Check sheet for the modelled part. Datum: model origin and axes. Units: mm. Face numbers are marked on the shaded views. A direction names the side the tool comes from. Coordinates: 2 decimals unless noted, no trailing zeros. Loops run counter-clockwise (first coordinate to the right, second up) from the corner with the lowest first, then second, coordinate; pieces in that order, holes last. Notation, with made-up numbers: M 81.25,55.25 L 98.25,55.25 A18 cw 98.25,68.25 Z; hole C -15,7 d5. An arc over 180 degrees is marked long. Return JSON: item names as keys, results as strings.
from build123d import *

# Parameters (mm, degrees)
SKETCH1_W                = 57.629592668
SKETCH1_H                = 21.211867522
SKETCH1_R                = 1.75
SKETCH1_R_2              = 4.5
BOSS_EXTRUDE1_DEPTH      = 6
SKETCH1_22_W             = 8.129592668
SKETCH1_22_H             = 21.211867522
SKETCH1_22_R             = 1.5
BOSS_EXTRUDE2_DEPTH      = 2
BOSS_EXTRUDE3_DEPTH      = 50.8
BOSS_EXTRUDE3_DEPTH_BACK = 50.8
SKETCH1_23_W             = 5
SKETCH1_23_H             = 75.291254256
SKETCH1_23_H_2           = 26.308745744
SKETCH4_W                = 57.748953374
SKETCH4_H                = 6
BOSS_EXTRUDE4_DEPTH      = 3
FILLET2_R                = 5
FILLET2_OF_MIRROR1_R     = 5


with BuildPart() as part:
    # Sketch1 → Boss-Extrude1 (new body)
    with BuildSketch(Plane(origin=(0, 0, 0), x_dir=(1, 0, 0), z_dir=(0, 1, 0))):
        with BuildLine():
            Line((-197.556308439, -13.154372872), (0, -13.154372872))
            ThreePointArc((0, -13.154372872), (13.154372872, 0), (0, 13.154372872))
            Line((0, 13.154372872), (-197.556308439, 13.154372872))
            Line((-197.556308439, 13.154372872), (-197.556308439, -13.154372872))
        make_face()
        with Locations((-104.57172107, -0.139435446)):
            Rectangle(SKETCH1_W, SKETCH1_H, mode=Mode.SUBTRACT)
        with Locations(Location((0, 8, 0), (0, 0, 270))):
            Circle(SKETCH1_R, mode=Mode.SUBTRACT)
        with Locations(Location((0, -8, 0), (0, 0, 270))):
            Circle(SKETCH1_R, mode=Mode.SUBTRACT)
        with Locations(Location((-8, 0, 0), (0, 0, 270))):
            Circle(SKETCH1_R, mode=Mode.SUBTRACT)
        with Locations(Location((0, 0, 0), (0, 0, 270))):
            Circle(SKETCH1_R_2, mode=Mode.SUBTRACT)
        with Locations(Location((8, 0, 0), (0, 0, 270))):
            Circle(SKETCH1_R, mode=Mode.SUBTRACT)
    boss_extrude1 = extrude(amount=BOSS_EXTRUDE1_DEPTH)

    # Sketch1<22> → Boss-Extrude2 (add)
    # profile 1 of 2: a face of its own
    with BuildSketch(Plane(origin=(0, 0, 0), x_dir=(1, 0, 0), z_dir=(0, 1, 0))):
        with Locations((-129.32172107, -0.139435446)):
            Rectangle(SKETCH1_22_W, SKETCH1_22_H)
        with Locations(Location((-129.32172107, -5, 0), (0, 0, 270))):
            Circle(SKETCH1_22_R, mode=Mode.SUBTRACT)
        with Locations(Location((-129.32172107, 5, 0), (0, 0, 270))):
            Circle(SKETCH1_22_R, mode=Mode.SUBTRACT)
    # profile 2 of 2: a face of its own
    with BuildSketch(Plane(origin=(0, 0, 0), x_dir=(1, 0, 0), z_dir=(0, 1, 0))):
        with Locations((-79.82172107, -0.139435446)):
            Rectangle(SKETCH1_22_W, SKETCH1_22_H)
        with Locations(Location((-79.82172107, -5, 0), (0, 0, 270))):
            Circle(SKETCH1_22_R, mode=Mode.SUBTRACT)
        with Locations(Location((-79.82172107, 5, 0), (0, 0, 270))):
            Circle(SKETCH1_22_R, mode=Mode.SUBTRACT)
    extrude(amount=BOSS_EXTRUDE2_DEPTH)

    # Sketch1<23> → Boss-Extrude3 (add, two sides: drawn at the far end of the back side and taken through both)
    with BuildSketch(Plane(origin=(0, 0, 0), x_dir=(1, 0, 0), z_dir=(0, 1, 0)).offset(-BOSS_EXTRUDE3_DEPTH_BACK)):
        with Locations((-200.056308439, 50.8)):
            Rectangle(SKETCH1_23_W, SKETCH1_23_H)
        with Locations((-200.056308439, 0)):
            Rectangle(SKETCH1_23_W, SKETCH1_23_H_2)
    extrude(amount=BOSS_EXTRUDE3_DEPTH + BOSS_EXTRUDE3_DEPTH_BACK)

    # Sketch4 → Boss-Extrude4 (add)
    with BuildSketch(Plane.XY.offset(13.154372872)):
        with Locations((-104.509525291, 3)):
            Rectangle(SKETCH4_W, SKETCH4_H)
    boss_extrude4 = extrude(amount=BOSS_EXTRUDE4_DEPTH)

    # Fillet2
    # the kernel refuses this fillet: 5 mm, written as the material it takes off along each edge
    with BuildSketch(Plane(origin=(-75.635048604, -11.456439237, 16.154372872), x_dir=(-1, 0, 0), z_dir=(0, 1, 0))) as fillet2_piece_1:
        with BuildLine():
            CenterArc((4.582575695, -5), FILLET2_R, 90, 66.421821522)
            Line((0, -3), (-0.091651514, -2.96))
            ThreePointArc((-0.091651514, -2.96), (-0.1, -1.5), (-0.1, 0))
            Line((-0.1, 0), (0, 0.1))
            Line((0, 0.1), (4.582575695, 0.1))
            Line((4.582575695, 0.1), (4.582575695, 0))
        make_face()
    extrude(amount=28.912878475, mode=Mode.SUBTRACT)
    with BuildSketch(Plane(origin=(-133.384001978, 17.456439237, 16.154372872), x_dir=(0, 0, -1), z_dir=(0, -1, 0))) as fillet2_piece_2:
        with BuildLine():
            CenterArc((5, 4.582575695), FILLET2_R, 180, 66.421821522)
            Line((0, 4.582575695), (-0.1, 4.582575695))
            Line((-0.1, 4.582575695), (-0.1, 0))
            Line((-0.1, 0), (0, -0.1))
            ThreePointArc((0, -0.1), (1.5, -0.1), (2.96, -0.091651514))
            Line((2.96, -0.091651514), (3, 0))
        make_face()
    extrude(amount=28.912878475, mode=Mode.SUBTRACT)

    # Mirror1: Boss-Extrude1, Boss-Extrude4 across plane
    add(boss_extrude1.mirror(Plane(origin=(0, 0, 0), x_dir=(1, 0, 0), z_dir=(0, 0, -1))))
    add(boss_extrude4.mirror(Plane(origin=(0, 0, 0), x_dir=(1, 0, 0), z_dir=(0, 0, -1))))

    # Fillet2 of Mirror1
    # the kernel refuses this fillet: 5 mm, written as the material it takes off along each edge
    with BuildSketch(Plane(origin=(-75.635048604, -11.456439237, -16.154372872), x_dir=(0, 0, 1), z_dir=(0, 1, 0)), Plane(origin=(-133.384001978, 17.456439237, -16.154372872), x_dir=(0, 0, 1), z_dir=(0, -1, 0))) as fillet2_of_mirror1_piece_1:
        with BuildLine():
            CenterArc((5, -4.582575695), FILLET2_OF_MIRROR1_R, 113.578178478, 66.421821522)
            Line((0, -4.582575695), (-0.1, -4.582575695))
            Line((-0.1, -4.582575695), (-0.1, 0))
            Line((-0.1, 0), (0, 0.1))
            ThreePointArc((0, 0.1), (1.5, 0.1), (2.96, 0.091651514))
            Line((2.96, 0.091651514), (3, 0))
        make_face()
    extrude(amount=28.912878475, mode=Mode.SUBTRACT)


solid = part.part
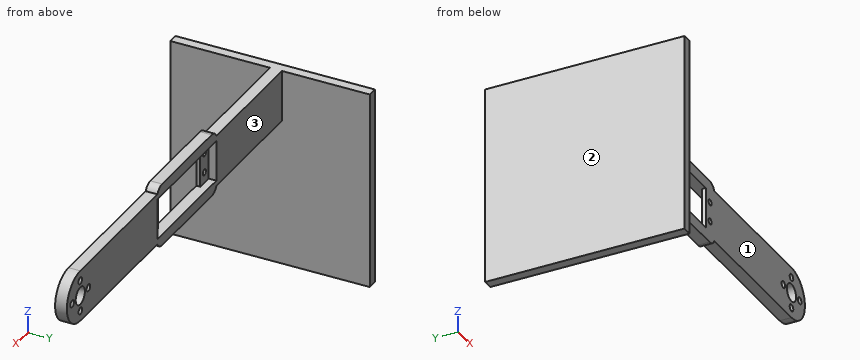
1) Section check B-B on y = -23.5. Record the cut outline in (x, z).
Answers:
{"outline": "M -202.56,-88.45 L -197.56,-88.45 L -197.56,13.15 L -202.56,13.15 Z"}
2) Section check C-C on x = -171.5. Record the cut outline in (y, z).
Answers:
{"outline": "M 0,-13.15 L 6,-13.15 L 6,13.15 L 0,13.15 Z"}
3) Scan lines: line 1 along X through (y, z) = (4.2, -8); line 2 along X through (y, z) = (4.2, 0); line 3 along X through (y, z) = (0.5, -0.5). Record each from-to range of solid material in increasing order. Write a range as [from, to].
Answers:
{"line 1": "[-202.56, -133.39], [-75.76, -1.75], [1.75, 10.44]", "line 2": "[-202.56, -133.39], [-75.76, -9.75], [-6.25, -4.5], [4.5, 6.25], [9.75, 13.15]", "line 3": "[-202.56, -125.26], [-83.89, -9.68], [-6.32, -4.47], [4.47, 6.32], [9.68, 13.14]"}
4) Set-up check for the marked faces 1, 2 and 3: record each of +Z, -Z, +X, -X, +Y, -Y from which the full face is reachable in a straight line by a thin tool's end or side.
Answers:
{"face 1": "+Z, -Z, +X, -Y", "face 2": "+Z, -Z, -X, +Y, -Y", "face 3": "+Z, -Z, +X, +Y"}
5) Go/stop test with flat-tipped pins: pin 1 Ø2 at (x, z) = (-162, -16) entering from -Y (1 decimal); pin 2 Ø3 at (y, z) = (-2.5, -38) entering from +X; pin 3 Ø16 at (x, z) = (-64, 1) entering from +Y; pin 4 Ø1.8 at (x, y) = (-36, 4) entering from +Z. Record where each tip stops, or that it passes through.
Answers:
{"pin 1": "through", "pin 2": "x = -197.56", "pin 3": "y = 6", "pin 4": "z = 13.15"}
6) Section check A-A on x = -91. Record the cut outline in (y, z).
Answers:
{"outline": "M 0,-16.15 L 6,-16.15 L 6,-10.47 L 0,-10.47 Z; M 0,10.47 L 6,10.47 L 6,16.15 L 0,16.15 Z"}
